Input: part model. Units: mm. Frame: model coordinates. Face numbers are marked on the shaded views. A direction names the side the tool comes from. Coordinates: 2 decimals unless noted, no trailing zeros. Order: outer loops, then holes, each group sorted by start corner. A loop starts at its lowest first (then second) coordinate and runs counter-clockwise, first axis right, second up. Notation, with made-up numbers: (24, -17.75) -> (63, -17.75) arc R17 ccw to (63, 0.25) -> close; hole circle Ø8 at (57.5, 33). An arc over 180 degrees is marked (long way). Answer as CSV lines item,"result".
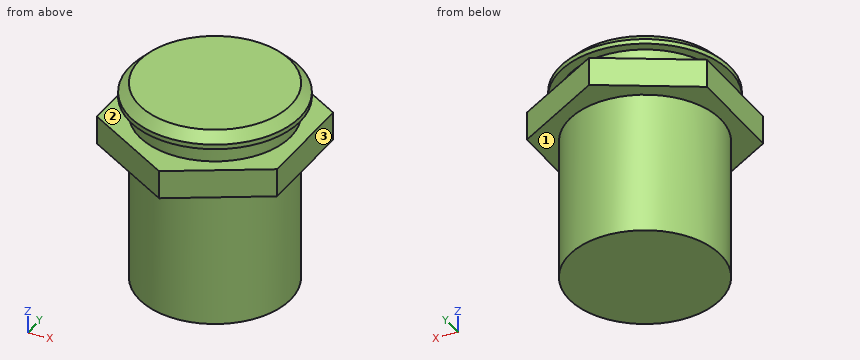
from build123d import *

# Parameters (mm, degrees)
F0_R     = 8
F1_DEPTH = 20
F0_R_2   = 9
F2_DEPTH = 1.5
F3_SIZE  = 1
F6_DEPTH = 3


with BuildPart() as f1:
    # F0 (on Top) → F1 (new body)
    with BuildSketch(Plane.XY):
        Circle(F0_R)
    extrude(amount=-F1_DEPTH)

    # F0 (on Top) → F2 (join)
    with BuildSketch(Plane.XY):
        Circle(F0_R_2)
        Circle(F0_R, mode=Mode.SUBTRACT)
        Circle(F0_R)
    extrude(amount=F2_DEPTH)

    # F3
    f3_edges = [f1.edges().sort_by_distance(p)[0] for p in [
        (-9, 0, 1.5),
    ]]
    chamfer(f3_edges, length=F3_SIZE)

    # F5 (on offset) → F6 (join)
    with BuildSketch(Plane.XY.offset(-2)):
        Polygon((9.5, 5.484828), (0, 10.969655), (-9.5, 5.484828), (-9.5, -5.484828), (0, -10.969655), (9.5, -5.484828), align=None)
    extrude(amount=-F6_DEPTH)


solid = f1.part
1. Cut plane B-B (z = -3.25). Return the cut outline in (x, y).
Findings:
outline,"(-9.5, -5.48) -> (0, -10.97) -> (9.5, -5.48) -> (9.5, 5.48) -> (0, 10.97) -> (-9.5, 5.48) -> close"
2. Cut plane A-A (y = 0). Return the cut outline in (x, z).
Findings:
outline,"(-9.5, -5) -> (-8, -5) -> (-8, -20) -> (8, -20) -> (8, -5) -> (9.5, -5) -> (9.5, -2) -> (8, -2) -> (8, 0) -> (9, 0) -> (9, 0.5) -> (8, 1.5) -> (-8, 1.5) -> (-9, 0.5) -> (-9, 0) -> (-8, 0) -> (-8, -2) -> (-9.5, -2) -> close"
3. Reachability of the marked faces 1, 2 and 3 from +Z, -Z, +X, -X, +Y, -Y: full face, straight path, thin tool, end or side. Return the list, or none.
Findings:
face 1,"-Z"
face 2,"none"
face 3,"+Z, -Z, +X, +Y, -Y"
4. Cut plane C-C (z = -16.5). Return the cut outline in (x, y).
Findings:
outline,"circle Ø16 at (0, 0)"
5. Contact query for flat-ended pins moving along their axis: pin 1 (8 mm diameter, centred on y = -6.5, z = -12, fed in from -X); pin 2 (1 mm diameter, centred on x = -4.5, z = -3, fed in from -Y); pin 3 (1.5 mm diameter, centred on x = -1, z = -11.5, fed in from +Y). Output: stop coordinate, or through.
Findings:
pin 1,"stops at x = -7.6"
pin 2,"stops at y = -8.66"
pin 3,"stops at y = 8"
6. Ray query, line 1 along Y through (x, z) = (-0.25, -6); line 2 along Z through (x, y) = (6.75, 5); line 3 along Y through (x, z) = (1.5, -6.5). Return the intervals inside material, ascending.
Findings:
line 1,"y = -8 to 8"
line 2,"z = -5 to -2, 0 to 1.1"
line 3,"y = -7.86 to 7.86"
